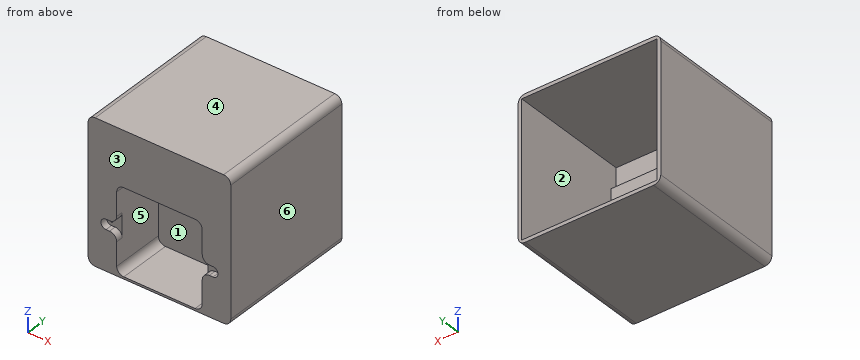
from build123d import *

# Parameters (mm, degrees)
SKETCH1_W             = 200
SKETCH1_H             = 200
BOSS_EXTRUDE1_DEPTH   = 200
SKETCH2_W             = 190
SKETCH2_H             = 190
CUT_EXTRUDE1_DEPTH    = 120
CUT_EXTRUDE2_DEPTH    = 75
CUT_EXTRUDE3_DEPTH    = 320
CUT_EXTRUDE4_DEPTH    = 50
CUT_EXTRUDE5_DEPTH    = 10
CROQUIS1_R            = 2.5
CORTAR_EXTRUIR1_DEPTH = 15
REDONDEO1_R           = 10


with BuildPart() as part:
    # Sketch1 → Boss-Extrude1 (new body)
    with BuildSketch(Plane(origin=(0, 0, 0), x_dir=(1, 0, 0), z_dir=(0, 1, 0))):
        Rectangle(SKETCH1_W, SKETCH1_H)
    extrude(amount=-BOSS_EXTRUDE1_DEPTH)

    # Sketch2 → Cut-Extrude1 (cut)
    with BuildSketch(Plane(origin=(0, 0, 0), x_dir=(1, 0, 0), z_dir=(0, 1, 0))):
        Rectangle(SKETCH2_W, SKETCH2_H)
    extrude(amount=-CUT_EXTRUDE1_DEPTH, mode=Mode.SUBTRACT)

    # Sketch3 → Cut-Extrude2 (cut)
    with BuildSketch(Plane(origin=(0, -200, 0), x_dir=(-1, 0, 0), z_dir=(0, -1, 0))):
        with BuildLine():
            Line((-60, 18.105219257), (-60, 87))
            ThreePointArc((-60, 87), (-57.071067812, 94.071067812), (-50, 97))
            Line((-50, 97), (50, 97))
            ThreePointArc((50, 97), (57.071067812, 94.071067812), (60, 87))
            Line((60, 87), (60, 18.105219257))
            Line((60, 18.105219257), (60, -13))
            ThreePointArc((60, -13), (57.071067812, -20.071067812), (50, -23))
            Line((50, -23), (-50, -23))
            ThreePointArc((-50, -23), (-57.071067812, -20.071067812), (-60, -13))
            Line((-60, -13), (-60, 18.105219257))
        make_face()
    extrude(amount=-CUT_EXTRUDE2_DEPTH, mode=Mode.SUBTRACT)

    # Sketch4 → Cut-Extrude3 (cut)
    with BuildSketch(Plane(origin=(0, -125, 0), x_dir=(-1, 0, 0), z_dir=(0, -1, 0))):
        with BuildLine():
            Line((11, -3.5), (-11, -3.5))
            ThreePointArc((-11, -3.5), (-11.5, -3), (-11, -2.5))
            Line((-11, -2.5), (11, -2.5))
            ThreePointArc((11, -2.5), (11.5, -3), (11, -3.5))
        make_face()
    extrude(amount=-CUT_EXTRUDE3_DEPTH, mode=Mode.SUBTRACT)

    # Sketch5 → Cut-Extrude4 (cut)
    with BuildSketch(Plane(origin=(0, -120, 0), x_dir=(1, 0, 0), z_dir=(0, 1, 0))):
        Polygon((-63, 95), (-63, -26), (63, -26), (63, 95), (95, 95), (95, -95), (-95, -95), (-95, 95), align=None)
    extrude(amount=-CUT_EXTRUDE4_DEPTH, mode=Mode.SUBTRACT)

    # Sketch6 → Cut-Extrude5 (cut)
    with BuildSketch(Plane.XZ.offset(200)):
        with BuildLine():
            Line((-70, -44), (-75, -44))
            ThreePointArc((-75, -44), (-82, -37), (-75, -30))
            Line((-75, -30), (-70, -30))
            ThreePointArc((-70, -30), (-62.928932188, -27.071067812), (-60, -20))
            Line((-60, -20), (-60, -54))
            ThreePointArc((-60, -54), (-62.928932188, -46.928932188), (-70, -44))
        make_face()
        with BuildLine():
            Line((70, -44), (75, -44))
            ThreePointArc((75, -44), (82, -37), (75, -30))
            Line((75, -30), (70, -30))
            ThreePointArc((70, -30), (62.928932188, -27.071067812), (60, -20))
            Line((60, -20), (60, -54))
            ThreePointArc((60, -54), (62.928932188, -46.928932188), (70, -44))
        make_face()
    extrude(amount=-CUT_EXTRUDE5_DEPTH, mode=Mode.SUBTRACT)

    # Croquis1 → Cortar-Extruir1 (cut)
    with BuildSketch(Plane.XZ.offset(190)):
        with Locations(Location((-75, -37, 0), (0, 0, 270))):
            Circle(CROQUIS1_R)
        with Locations(Location((75, -37, 0), (0, 0, 90))):
            Circle(CROQUIS1_R)
    extrude(amount=-CORTAR_EXTRUIR1_DEPTH, mode=Mode.SUBTRACT)

    # Redondeo1
    redondeo1_edges = [part.edges().sort_by_distance(p)[0] for p in [
        (100, -100, 100),
        (-100, -100, 100),
        (-100, -100, -100),
        (100, -100, -100),
    ]]
    fillet(redondeo1_edges, radius=REDONDEO1_R)


solid = part.part
Design review of the part built by this model. Coordinates are the model's own, in mm. Face numbers are marked on the shaded views. A direction names the side the tool comes from. Coordinates: 2 decimals unless noted, no trailing zeros. Loops run counter-clockwise (first coordinate to the right, second up) from the corner with the lowest first, then second, coordinate; pieces in that order, holes last. Notation, with made-up numbers: (32.25, 49.25) - (47.25, 49.25) arc R27 ccw to (47.25, 73.25) - close; hole circle Ø5 at (-39, 64.25). An arc over 180 degrees is marked (long way). Use CSV: the item, a comma, the result in double quotes. Start each with the question number.
1. Add section D-D on z = 19.5. Give the boundary of the cut face in (x, y), plus the area to 3 significant figures.
2. For the marked faces 1, 2 and 3, list the 3-axis set-ups (+Z, -Z, +X, -X, +Y, -Y) from which the entire face can be reached by the end or side of a thin tool; tool diameter is ignored.
3. Mouldability with a two-part tool opening along X and no side actions: class the marked faces 4, 5 and 6 as released by +X, released by -X, zero draft, split by the parting line, or undercut.
4. Add section A-A on z = 47. Give the boundary of the cut face in (x, y), plus the area to 3 significant figures.
5. Add section B-B on y = -14. Give the boundary of the cut face in (x, z).
6. Clearance check with flat-ended pins moving along their axes: pin 1 (4 mm diameter, centred on x = -12.5, z = -62, fed in from -Y); pin 2 (8 mm diameter, centred on x = -75, z = -37, fed in from -Y); pin 3 (8 mm diameter, centred on x = 38.5, z = -78, fed in from +Y). State where each tip first meets the part, or that it passes through.
7. To check wall thickness, follow probe 1 along X at (y, z) = (-183, -37); probe 2 along X at (y, z) = (-135, -15.5); probe 3 along Z at (x, y) = (-57.5, -20). State the ranges of each line that lie inside material, in increasing order.
8. Add section C-C on x = 14.5. Give the boundary of the cut face in (y, z).
Resolved:
1,outline,"(-100, -200) - (-57.6, -200) - (-57.6, -125) - (57.6, -125) - (57.6, -200) - (100, -200) - (100, 0) - (95, 0) - (95, -170) - (63, -170) - (63, -120) - (-63, -120) - (-63, -170) - (-95, -170) - (-95, 0) - (-100, 0) - close"
1,area,"5,360 mm2"
2,face 1,"-Y"
2,face 2,"+Y"
2,face 3,"+Z, -Z, +X, -X, -Y"
3,face 4,"zero draft"
3,face 5,"undercut"
3,face 6,"released by +X"
4,outline,"(-100, -200) - (100, -200) - (100, 0) - (95, 0) - (95, -170) - (-95, -170) - (-95, 0) - (-100, 0) - close"
4,area,"7,700 mm2"
5,outline,"(-100, -90) arc R10 ccw to (-90, -100) - (90, -100) arc R10 ccw to (100, -90) - (100, 90) arc R10 ccw to (90, 100) - (-90, 100) arc R10 ccw to (-100, 90) - close; hole (-95, -95) - (95, -95) - (95, 95) - (-95, 95) - close"
6,pin 1,"y = -125"
6,pin 2,"y = -190"
6,pin 3,"y = -120"
7,probe 1,"-100 to -77.5, -72.5 to -60, 60 to 72.5, 77.5 to 100"
7,probe 2,"-100 to -95, -63 to -60, 60 to 63, 95 to 100"
7,probe 3,"-100 to -95, 95 to 100"
8,outline,"(-200, -100) - (0, -100) - (0, -95) - (-120, -95) - (-120, 26) - (-170, 26) - (-170, 95) - (0, 95) - (0, 100) - (-200, 100) - (-200, 23) - (-125, 23) - (-125, -97) - (-200, -97) - close"
